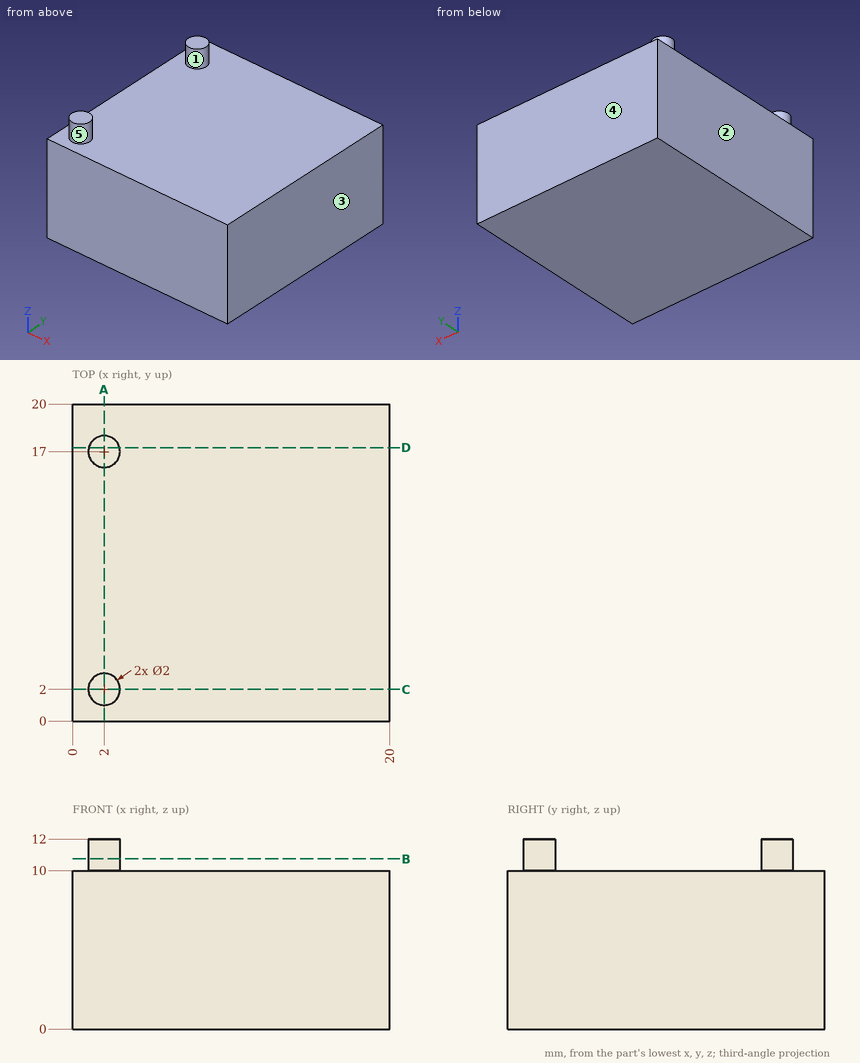
Here's the drawing with two shaded views (mm, measured from the low corner). I have some questions. A direction names the side the tool comes from. Round coordinates to 2 decimals unless told otherwise and drop trailing zeros. Loops run counter-clockwise (first coordinate to the right, second up) from the corner with the lowest first, then second, coordinate; pieces in that order, holes last.
Item 1: Suppose I cut it at A-A, the plane x = 2. Write out the boundary of the cut face in (y, z), then the cut area to 3 significant figures.
Item 2: Suppose I cut it at C-C, the plane y = 2. Write out the boundary of the cut face in (x, z), then the cut area to 3 significant figures.
Item 3: Suppose I cut it at D-D, the plane y = 17.25. Write out the boundary of the cut face in (x, z), then the cut area to 3 significant figures.
Item 4: If we mould it in two halves opening along Y, with no side actions, what happens to the marked faces 3, 4 and 5? For each: +Y half, -Y half, draft (parallel to the pull), parting line (faces both ways), or undercut.
Item 5: Suppose I cut it at B-B, the plane z = 10.75. Write out the boundary of the cut face in (x, y).
Item 6: Please list where this line runs through material, in increasing order: L1, parallel to Z at x = 11.25, y = 4.5.
Item 7: Which directions (+Z, -Z, +X, -X, +Y, -Y) give clear straight access to the entire face, cutting with the end or side of a thin tool? Please do the marked faces 1 and 2.
Reported:
1. outline: (0, 0) - (20, 0) - (20, 10) - (18, 10) - (18, 12) - (16, 12) - (16, 10) - (3, 10) - (3, 12) - (1, 12) - (1, 10) - (0, 10) - close
1. area: 208 mm2
2. outline: (0, 0) - (20, 0) - (20, 10) - (3, 10) - (3, 12) - (1, 12) - (1, 10) - (0, 10) - close
2. area: 204 mm2
3. outline: (0, 0) - (20, 0) - (20, 10) - (2.97, 10) - (2.97, 12) - (1.03, 12) - (1.03, 10) - (0, 10) - close
3. area: 204 mm2
4. face 3: draft
4. face 4: +Y half
4. face 5: undercut
5. outline: circle Ø2 at (2, 2); circle Ø2 at (2, 17)
6. L1: z = 0 to 10
7. face 1: +Z
7. face 2: +Z, -Z, -X, +Y, -Y
